Here's how the part is built. I have some questions about the finished solid (model axes, mm). Round coordinates to 2 decimals unless told otherwise and drop trailing zeros. Order: outer loops, then holes, each group sorted by start corner. A loop starts at its lowest first (then second) coordinate and runs counter-clockwise, first axis right, second up. Notation, with made-up numbers: (74, -29.5) - (84, -29.5) arc R13 cw to (84, -9.5) - close; hole circle Ø11 at (8.5, 3). An arc over 180 degrees is marked (long way). Answer as a JSON object with one key per item and string values.
```python
from build123d import *
from build123d.topology import SkipClean

# Parameters (mm, degrees)
SKETCH1_R           = 4
BOSS_EXTRUDE1_DEPTH = 35
CUT_EXTRUDE1_DEPTH  = 22
SKETCH3_R           = 2.5
CUT_EXTRUDE2_DEPTH  = 4
SKETCH4_W           = 3
SKETCH4_H           = 3
CUT_EXTRUDE3_DEPTH  = 5


with BuildPart() as part:
    # Sketch1 → Boss-Extrude1 (new body)
    with BuildSketch(Plane(origin=(0, 0, 0), x_dir=(1, 0, 0), z_dir=(0, 1, 0))):
        with Locations(Location((0, 0, 0), (0, 0, 270))):
            Circle(SKETCH1_R)
    extrude(amount=BOSS_EXTRUDE1_DEPTH)

    # Sketch2 → Cut-Extrude1 (cut)
    with BuildSketch(Plane.XZ):
        with BuildLine():
            Line((-1.5, 2), (1.5, 2))
            ThreePointArc((1.5, 2), (0, -2.5), (-1.5, 2))
        make_face()
    extrude(amount=-CUT_EXTRUDE1_DEPTH, mode=Mode.SUBTRACT)

    # Sketch3 → Cut-Extrude2 (cut)
    with SkipClean():  # the faces are left unmerged after this step: merging them gives an invalid solid
        with BuildSketch(Plane.XZ):
            with Locations(Location((0, 0, 0), (0, 0, 270))):
                Circle(SKETCH3_R)
        extrude(amount=-CUT_EXTRUDE2_DEPTH, mode=Mode.SUBTRACT)

    # Sketch4 → Cut-Extrude3 (cut)
    with SkipClean():  # the faces are left unmerged after this step: merging them gives an invalid solid
        with BuildSketch(Plane(origin=(0, 35, 0), x_dir=(1, 0, 0), z_dir=(0, 1, 0))):
            with Locations((-4, 0)):
                Rectangle(SKETCH4_W, SKETCH4_H)
        extrude(amount=-CUT_EXTRUDE3_DEPTH, mode=Mode.SUBTRACT)


solid = part.part
```
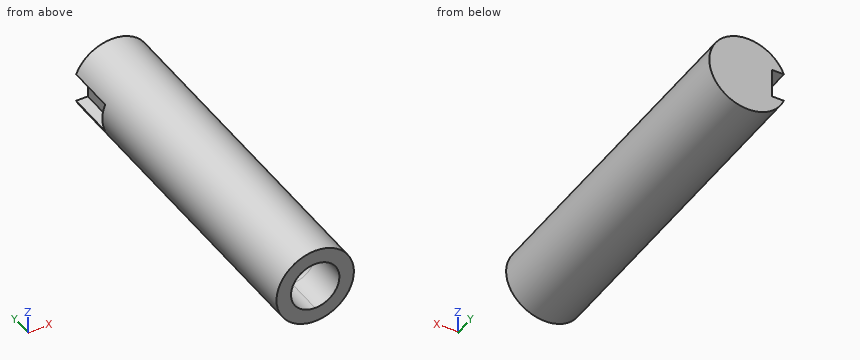
1. If I drill on L1, parallel to Z at x = 0, y = 16; L2, parallel to X at y = 15.5, z = 0; L3, parallel to Y at x = -1.25, z = -0.25, over which ranges is the centre line in solid material (lowest first)? Write a range as [from, to].
Responses:
{"L1": "[-4, -2.5], [2, 4]", "L2": "[-4, -2.5], [2.5, 4]", "L3": "[22, 35]"}
2. Imagine slicing it at C-C (y = 29). List the corners of the cut face in (x, z) for me.
Responses:
{"outline": "circle Ø8 at (0, 0)"}
3. Imagine slicing it at B-B (x = -2). List the corners of the cut face in (y, z) for me, plus the area to 3 significant figures.
Responses:
{"outline": "(0, -3.46) - (35, -3.46) - (35, 3.46) - (0, 3.46) - (0, 1.5) - (22, 1.5) - (22, -1.5) - (0, -1.5) - close", "area": "176 mm2"}
4. Imagine slicing it at A-A (z = 0). List the corners of the cut face in (x, y) for me.
Responses:
{"outline": "(-4, 0) - (-2.5, 0) - (-2.5, 22) - (2.5, 22) - (2.5, 0) - (4, 0) - (4, 35) - (-2.5, 35) - (-2.5, 30) - (-4, 30) - close"}
5. Imagine slicing it at D-D (z = -2). List the corners of the cut face in (x, y) for me.
Responses:
{"outline": "(-3.46, 0) - (-1.5, 0) - (-1.5, 22) - (1.5, 22) - (1.5, 0) - (3.46, 0) - (3.46, 35) - (-3.46, 35) - close"}
6. For P1, Ø0.8, axis at x = -3.5, z = 0.5, coming from the +Y side; P2, Ø2, axis at x = 0.5, z = -0.5, coming from the -Y side; P3, Ø1, axis at x = -3.5, y = 33, coming from the -Z side, each with a flat end and sliding along its axis, tell me the tip position at first contact or that it passes through.
Responses:
{"P1": "y = 30", "P2": "y = 22", "P3": "z = -2.65"}
